Verification items for the finished model (mm, model axes). Coordinates: 2 decimals unless noted, no trailing zeros. Order: outer loops, then holes, each group sorted by start corner. A loop starts at its lowest first (then second) coordinate and runs counter-clockwise, first axis right, second up.
Q1. Draft check along Z on faces 1 (the cylindrical face through (-12, 1, 0)), 2 (the cylindrical face through (0.07, 1.48, -21.5)), 3 (the flat face through (-12.195, 1.479, -15.726)), 4 (the flat face through (-4, 0, 0)). Enter one of: pulls with the +Z half, pulls with the -Z half, needs draft (parallel to the pull), parting line crosses it, or undercut.
Q2. Cross-section at A-A, the plane z = 0. Record the boundary of the cut face in (x, y), and give its area (3 significant figures).
Q3. Cross-section at C-C, the plane x = 0. Record the boundary of the cut face in (y, z), and give its area (3 significant figures).
Q4. Depth check by flat-ended pin: P1, Ø2.5, axis at x = -10.5, z = 0, coming from the -Y side. Enter the tip coordinate at first touch or a pass-through.
Q5. Cross-section at B-B, the plane y = 1.55. Record the boundary of the cut face in (x, z).
Q6. Thickness scan on line 1 (X direction, y = 1, z = 0); line 2 (X direction, y = 0.7, z = 21); line 3 (X direction, y = 0.95, z = 15). Record the ranges inside material, lowest first.
Q7. Cross-section at D-D, the plane x = -11. Record the boundary of the cut face in (y, z).
from build123d import *

# Parameters (mm, degrees)
SKETCH_1_R      = 1.5
EXTRUDE_1_DEPTH = 3


with BuildPart() as part:
    # ｽｹｯﾁ1 → ﾎﾞｽ - 押し出し1 (new body)
    with BuildSketch(Plane(origin=(0, 0, 0), x_dir=(1, 0, 0), z_dir=(0, 1, 0))):
        with BuildLine():
            Line((6.5, 20), (6.5, 0))
            Line((6.5, 0), (6.5, -20))
            ThreePointArc((6.5, -20), (2.24911051, -26.098483575), (-4.94353905, -24.220358001))
            Line((-4.94353905, -24.220358001), (-19.246261396, -7.466787233))
            ThreePointArc((-19.246261396, -7.466787233), (-22, 0), (-19.246261396, 7.466787233))
            Line((-19.246261396, 7.466787233), (-4.94353905, 24.220358001))
            ThreePointArc((-4.94353905, 24.220358001), (2.24911051, 26.098483575), (6.5, 20))
        make_face()
        with Locations(Location((0, 0, 0), (0, 0, 270))):
            Circle(SKETCH_1_R, mode=Mode.SUBTRACT)
        with Locations(Location((0, 20, 0), (0, 0, 270))):
            Circle(SKETCH_1_R, mode=Mode.SUBTRACT)
        with Locations(Location((0, -20, 0), (0, 0, 270))):
            Circle(SKETCH_1_R, mode=Mode.SUBTRACT)
        with Locations(Location((-10.5, 0, 0), (0, 0, 270))):
            Circle(SKETCH_1_R, mode=Mode.SUBTRACT)
    extrude(amount=EXTRUDE_1_DEPTH)


solid = part.part
Check values:
1. face 1: undercut
1. face 2: undercut
1. face 3: pulls with the -Z half
1. face 4: needs draft
2. outline: (-22, 0) - (-12, 0) - (-12, 3) - (-22, 3) - close; (-9, 0) - (-1.5, 0) - (-1.5, 3) - (-9, 3) - close; (1.5, 0) - (6.5, 0) - (6.5, 3) - (1.5, 3) - close
2. area: 67.5 mm2
3. outline: (0, -26.5) - (3, -26.5) - (3, -21.5) - (0, -21.5) - close; (0, -18.5) - (3, -18.5) - (3, -1.5) - (0, -1.5) - close; (0, 1.5) - (3, 1.5) - (3, 18.5) - (0, 18.5) - close; (0, 21.5) - (3, 21.5) - (3, 26.5) - (0, 26.5) - close
3. area: 132 mm2
4. P1: passes through
5. outline: (-19.25, -7.47) - (-4.94, -24.22) arc R6.5 ccw to (6.5, -20) - (6.5, 20) arc R6.5 ccw to (-4.94, 24.22) - (-19.25, 7.47) arc R11.5 ccw to start; hole circle Ø3 at (-10.5, 0); hole circle Ø3 at (0, -20); hole circle Ø3 at (0, 0); hole circle Ø3 at (0, 20)
6. line 1: x = -22 to -12, -9 to -1.5, 1.5 to 6.5
6. line 2: x = -7.69 to -1.12, 1.12 to 6.42
6. line 3: x = -12.82 to 6.5
7. outline: (0, -17.13) - (3, -17.13) - (3, -1.41) - (0, -1.41) - close; (0, 1.41) - (3, 1.41) - (3, 17.13) - (0, 17.13) - close
